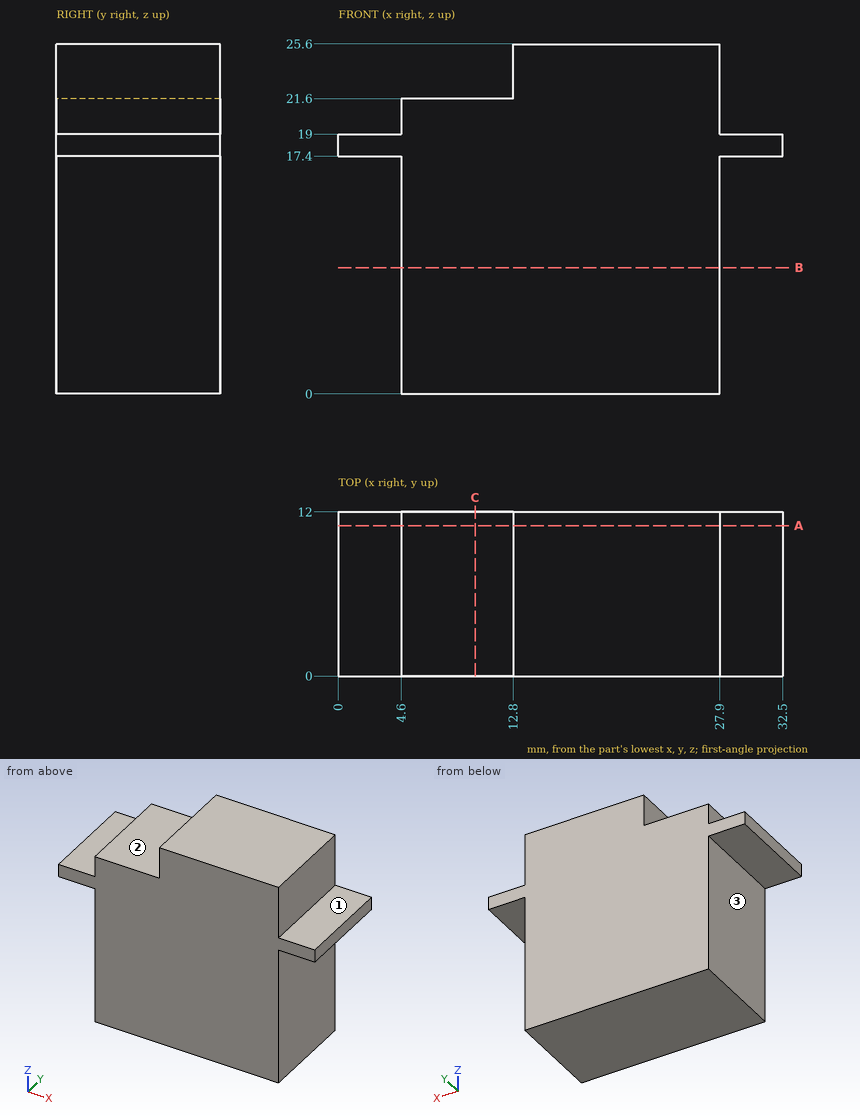
Geometry check sheet. Reference: drawing and pictorial views, mm from the part's lowest x, y, z. A direction names the side the tool comes from. Give positions to 0.01 mm unless a question says otherwise; leave off trailing zeros. Order: outer loops, then holes, each group sorted by start corner. A loop starts at its lowest first (then second) coordinate and runs counter-clockwise, first axis right, second up. Notation, with made-up numbers: (-29.75, 24) - (0.25, 24) arc R9 cw to (0.25, 35) - close; hole circle Ø6 at (31.25, 46). An arc over 180 degrees is marked (long way). Answer as CSV lines item,"result". Start each with the question number.
Item 1: Section check B-B, the plane z = 9.25. Record the boundary of the cut face in (x, y).
Item 2: Section check C-C, the plane x = 10. Record the boundary of the cut face in (y, z), plus the area to 3 significant figures.
Item 3: Gauge pin test, flat ends, axial feed: pin 1 (1.2 mm diameter, centred on y = 8, z = 24, fed in from -X); pin 2 (2.5 mm diameter, centred on x = 29.5, y = 3, fed in from -Z); pin 3 (2.5 mm diameter, centred on x = 2, y = 4.5, fed in from +Z). Record the tip position at first contact, or that the pin passes through.
Item 4: Access from +Z, -Z, +X, -X, +Y, -Y to the whole of each face (thin tool, end or side, straight path). Record for the marked faces 1, 2 and 3.
Item 5: Section check A-A, the plane y = 11. Record the boundary of the cut face in (x, z), plus the area to 3 significant figures.
Item 6: Material ranges on L1, parallel to X at y = 1.5, z = 9.75; L2, parallel to Z at x = 29, y = 5.5; L3, parallel to X at y = 7.5, z = 24.25, recorded low to high.
Filled in:
1,outline,"(4.6, 0) - (27.9, 0) - (27.9, 12) - (4.6, 12) - close"
2,outline,"(0, 0) - (12, 0) - (12, 21.6) - (0, 21.6) - close"
2,area,"259 mm^2"
3,pin 1,"x = 12.8"
3,pin 2,"z = 17.4"
3,pin 3,"z = 19"
4,face 1,"+Z, +X, +Y, -Y"
4,face 2,"+Z, -X, +Y, -Y"
4,face 3,"-Z, -X, +Y, -Y"
5,outline,"(0, 17.4) - (4.6, 17.4) - (4.6, 0) - (27.9, 0) - (27.9, 17.4) - (32.5, 17.4) - (32.5, 19) - (27.9, 19) - (27.9, 25.6) - (12.8, 25.6) - (12.8, 21.6) - (4.6, 21.6) - (4.6, 19) - (0, 19) - close"
5,area,"578 mm^2"
6,L1,"4.6 to 27.9"
6,L2,"17.4 to 19"
6,L3,"12.8 to 27.9"
